Read the model definition and answer for the solid it produces. Units are mm, in the model's axes. Face numbers are marked on the shaded views. A direction names the side the tool comes from. Coordinates: 2 decimals unless noted, no trailing zeros. Order: outer loops, then holes, each group sorted by start corner. A loop starts at its lowest first (then second) coordinate and runs counter-clockwise, first axis right, second up. Notation, with made-up numbers: (38.25, -28.5) -> (92.25, -28.5) arc R8 ccw to (92.25, -15.5) -> close; hole circle Ø5 at (56.25, 23). An arc over 180 degrees is marked (long way). Answer in a Markdown table with one row per item.
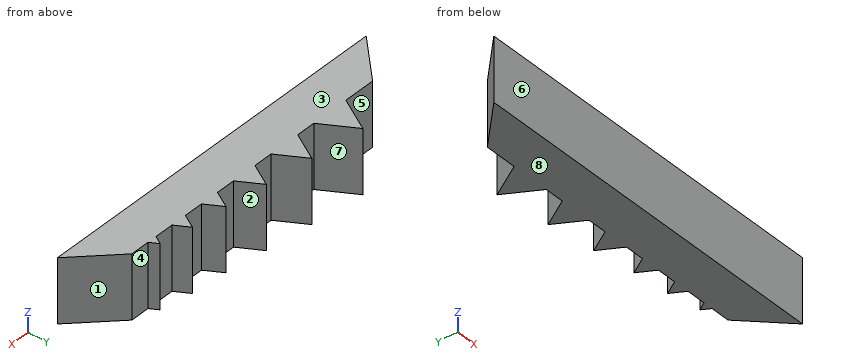
from build123d import *

# Parameters (mm, degrees)
F1_DEPTH = 100


with BuildPart() as f1:
    # F0 (on Top) → F1 (new body)
    with BuildSketch(Plane.XY):
        Polygon((-63.63961, -513.63961), (513.63961, -513.63961), (450, -450), (420, -450), (405, -450), (375, -450), (350, -450), (320, -450), (290, -450), (260, -450), (220, -450), (190, -450), (140, -450), (110, -450), (50, -450), (0, -450), align=None)
        Polygon((80, -398.038476), (50, -450), (110, -450), align=None)
        Polygon((165, -406.69873), (140, -450), (190, -450), align=None)
        Polygon((240, -415.358984), (220, -450), (260, -450), align=None)
        Polygon((290, -450), (320, -450), (305, -424.019238), align=None)
        Polygon((350, -450), (375, -450), (362.5, -428.349365), align=None)
        Polygon((405, -450), (420, -450), (412.5, -437.009619), align=None)
    extrude(amount=F1_DEPTH)


solid = f1.part
Q1. Given pin 1 (15 mm diameter, centred on x = 395.5, z = 56, fed in from +Y); pin 2 (1 mm diameter, centred on x = 306.5, z = 62, fed in from +Y); pin 3 (10 mm diameter, centred on y = -436, z = 54, fed in from +X), each flat-ended and moving along its own axis, determine where each tip first touches the part or whether it passes through.
Outcome:
| item | result |
|---|---|
| pin 1 | y = -450 |
| pin 2 | y = -425.75 |
| pin 3 | x = 414.8 |
Q2. The part is cut by section C-C (x = 28). Write down the section's boundary in (y, z).
Outcome:
| item | result |
|---|---|
| outline | (-513.64, 0) -> (-450, 0) -> (-450, 100) -> (-513.64, 100) -> close |
Q3. For the marked faces 4, 5, 6, 7 and 8, determine the directions among +Z, -Z, +X, -X, +Y, -Y from which every point of the face is accessible in a straight line to the end or side of a thin tool.
Outcome:
| item | result |
|---|---|
| face 4 | +Z, -Z, +X, +Y |
| face 5 | +Z, -Z, -X, +Y |
| face 6 | +Z, -Z, +X, -X, -Y |
| face 7 | +Z, -Z, +Y |
| face 8 | -Z, +X, -X, +Y, -Y |
Q4. Consider line 1 (X direction, y = -430, z = 33); line 2 (X direction, y = -423, z = 24.5); line 3 (X direction, y = -441.5, z = 14.5). Determine where each line is inside the solid, lowest interval first.
Outcome:
| item | result |
|---|---|
| line 1 | 61.55 to 98.45, 151.55 to 178.45, 231.55 to 248.45, 301.55 to 308.45, 361.55 to 363.45 |
| line 2 | 65.59 to 94.41, 155.59 to 174.41, 235.59 to 244.41 |
| line 3 | 54.91 to 105.09, 144.91 to 185.09, 224.91 to 255.09, 294.91 to 315.09, 354.91 to 370.09, 409.91 to 415.09 |
Q5. The part is cut by section B-B (y = -506). Write down the section's boundary in (x, z), then the cut area to 3 significant figures.
Outcome:
| item | result |
|---|---|
| outline | (-56, 0) -> (506, 0) -> (506, 100) -> (-56, 100) -> close |
| area | 56,200 mm² |
Q6. For a pull along X with two mould halves and no side action, classify the marked faces 1, 2 and 3 as pulls with the +X half, pulls with the -X half, needs draft (parallel to the pull), parting line crosses it, or undercut.
Outcome:
| item | result |
|---|---|
| face 1 | pulls with the +X half |
| face 2 | undercut |
| face 3 | needs draft |
Q7. The part is cut by section A-A (z = 20). Write down the section's boundary in (x, y).
Outcome:
| item | result |
|---|---|
| outline | (-63.64, -513.64) -> (513.64, -513.64) -> (450, -450) -> (420, -450) -> (412.5, -437.01) -> (405, -450) -> (375, -450) -> (362.5, -428.35) -> (350, -450) -> (320, -450) -> (305, -424.02) -> (290, -450) -> (260, -450) -> (240, -415.36) -> (220, -450) -> (190, -450) -> (165, -406.7) -> (140, -450) -> (110, -450) -> (80, -398.04) -> (50, -450) -> (0, -450) -> close |
